Work out the finished part from the listing and answer in its coordinate system (mm). A direction names the side the tool comes from. Coordinates: 2 decimals unless noted, no trailing zeros. Order: outer loops, then holes, each group sorted by start corner. A loop starts at its lowest first (then second) coordinate and runs counter-clockwise, first axis right, second up. Notation, with made-up numbers: M 49.25,73 L 108.25,73 A13 cw 108.25,97 Z; hole C 85,-22 d2. An arc over 180 degrees is marked long. Use a Markdown table: item, result.
from build123d import *

# Parameters (mm, degrees)
F1_DEPTH       = 7
F3_DEPTH       = 3
F4_D           = 3.5
F5_R           = 1
F7_D           = 3.5
F7_CBORE_D     = 5.6
F7_CBORE_DEPTH = 2.1


# Not quite as in the source:
# - a feature names something its author has since deleted; it is built from what else it names


with BuildPart() as f1:
    # F0 (on Top) → F1 (new body)
    with BuildSketch(Plane.XY):
        with BuildLine():
            Line((48.5705398023, 9.4616535902), (-39.4294601977, 9.4616535902))
            Line((-39.4294601977, 9.4616535902), (-39.4294601977, -5.5383464098))
            Line((-39.4294601977, -5.5383464098), (-34.5486067235, -5.5383464098))
            Line((-34.5486067235, -5.5383464098), (-34.5486067235, -5.0383464098))
            ThreePointArc((-34.5486067235, -5.0383464098), (-33.3770338483, -2.2099192851), (-30.5486067235, -1.0383464098))
            Line((-30.5486067235, -1.0383464098), (-9.5486067235, -1.0383464098))
            ThreePointArc((-9.5486067235, -1.0383464098), (-6.7201795988, -2.2099192851), (-5.5486067235, -5.0383464098))
            Line((-5.5486067235, -5.0383464098), (-5.5486067235, -5.5383464098))
            Line((-5.5486067235, -5.5383464098), (14.3895465881, -5.5383464098))
            Line((14.3895465881, -5.5383464098), (14.3895465881, -5.0383464098))
            ThreePointArc((14.3895465881, -5.0383464098), (15.5611194633, -2.2099192851), (18.3895465881, -1.0383464098))
            Line((18.3895465881, -1.0383464098), (39.3895465881, -1.0383464098))
            ThreePointArc((39.3895465881, -1.0383464098), (42.2179737128, -2.2099192851), (43.3895465881, -5.0383464098))
            Line((43.3895465881, -5.0383464098), (43.3895465881, -6.5383464098))
            Line((43.3895465881, -6.5383464098), (48.5705398023, -6.5383464098))
            Line((48.5705398023, -6.5383464098), (48.5705398023, 9.4616535902))
        make_face()
    extrude(amount=F1_DEPTH)

    # F2 (on face) → F3 (cut)
    with BuildSketch(Plane.XY.offset(7)):
        Polygon((17.7705398023, 0.1141327288), (17.7705398023, 3.8091744516), (14.5705398023, 5.656695313), (11.3705398023, 3.8091744516), (11.3705398023, 0.1141327288), (14.5705398023, -1.7333881326), align=None)
        Polygon((-8.6294601977, 3.8091744516), (-8.6294601977, 0.1141327288), (-5.4294601977, -1.7333881326), (-2.2294601977, 0.1141327288), (-2.2294601977, 3.8091744516), (-5.4294601977, 5.656695313), align=None)
    extrude(amount=-F3_DEPTH, mode=Mode.SUBTRACT)

    # F4 (through all)
    with Locations(Plane.XY.offset(7)):
        with Locations((-5.4294601977, 1.9616535902), (14.5705398023, 1.9616535902)):
            Hole(F4_D / 2)

    # F5
    f5_edges = [f1.edges().sort_by_distance(p)[0] for p in [
        (48.57054, 1.461654, 0),
        (4.57054, 9.461654, 0),
        (-39.42946, 1.961654, 0),
    ]]
    fillet(f5_edges, radius=F5_R)

    # F7 (through all)
    with Locations(Plane(origin=(0, 0, 0), x_dir=(1, 0, 0), z_dir=(0, 0, -1))):
        with Locations((-34.4294601977, -1.9616535902), (43.5705398023, -1.9616535902)):
            CounterBoreHole(F7_D / 2, F7_CBORE_D / 2, F7_CBORE_DEPTH)


solid = f1.part
1. Section A-A on y = -3 is taken. Determine the outline of the cut face in (x, z), then the cut area to 3 significant figures.
Answers below:
| item | result |
|---|---|
| outline | M -39.43,1 A1 ccw -38.43,0 L -33.99,0 L -33.99,7 L -39.43,7 Z; M -6.11,0 L 14.95,0 L 14.95,7 L -6.11,7 Z; M 42.83,0 L 47.57,0 A1 ccw 48.57,1 L 48.57,7 L 42.83,7 Z |
| area | 225 mm² |
2. Flat-ended cylindrical pins translate along their axes: P1, Ø1.9, axis at x = -6, y = 3, coming from the +Z side; P2, Ø3.5, axis at x = 7.5, z = 3, coming from the -Y side; P3, Ø3, axis at x = -5.43, y = 1.96, coming from the -Z side; P4, Ø3, axis at x = -34, y = 2.5, coming from the -Z side. Find the tip coordinate at first contact, or state that the pin passes through.
Answers below:
| item | result |
|---|---|
| P1 | z = 4 |
| P2 | y = -5.54 |
| P3 | through |
| P4 | z = 2.1 |
3. For faces 1 (the face through (12.993, 4.746, 5.521)), 2 (the face through (43.39, -6, 3)), 3 (the face through (-36.65, 3.67, 1.04)), determine the directions among +Z, -Z, +X, -X, +Y, -Y from which every point of the face is accessible in a straight line to the end or side of a thin tool.
Answers below:
| item | result |
|---|---|
| face 1 | +Z |
| face 2 | +Z, -Z, -Y |
| face 3 | -Z |
4. Section D-D on x = 5 is taken. Determine the outline of the cut face in (y, z), then the cut area to 3 significant figures.
Answers below:
| item | result |
|---|---|
| outline | M -5.54,0 L 8.46,0 A1 ccw 9.46,1 L 9.46,7 L -5.54,7 Z |
| area | 105 mm² |
5. Section B-B on x = 36 is taken. Determine the outline of the cut face in (y, z).
Answers below:
| item | result |
|---|---|
| outline | M -1.04,0 L 8.46,0 A1 ccw 9.46,1 L 9.46,7 L -1.04,7 Z |
6. Find the intervals of material crossed by probe 1 along X at (y, z) = (-5, 1); probe 2 along X at (y, z) = (1.75, 1.25); probe 3 along X at (y, z) = (-2.5, 1.5), in increasing order.
Answers below:
| item | result |
|---|---|
| probe 1 | -39.43 to -34.55, -5.55 to 14.39, 43.39 to 48.57 |
| probe 2 | -39.43 to -37.22, -31.64 to -7.17, -3.69 to 12.83, 16.31 to 40.78, 46.36 to 48.57 |
| probe 3 | -39.43 to -33.64, -6.46 to 15.3, 42.48 to 48.57 |
7. Section C-C on z = 5 is taken. Give the number of separate pieces and of enclosed holes in the cut face, then the cut area to 3 significant figures.
Answers below:
| item | result |
|---|---|
| separate pieces | 1 |
| enclosed holes | 4 |
| area | 988 mm² |
